CAD build for the part. Positions are in the model's coordinates, mm. A direction names the side the tool comes from. Coordinates: 2 decimals unless noted, no trailing zeros. Write each loop counter-clockwise with the first axis right and the second up, starting at its lowest first coordinate (ties: lowest second). Pieces come first, ordered by that corner, then holes. Notation, with made-up numbers: (67, 68) -> (126, 68) arc R13 cw to (126, 82) -> close; hole circle Ø10 at (26.25, -28). An arc over 180 degrees is marked (long way). Answer as CSV lines item,"result".
```python
from build123d import *

# Parameters (mm, degrees)
SKETCH1_W               = 38.1
SKETCH1_H               = 152.4
BOSS_EXTRUDE1_DEPTH     = 12.7
FILLET1_R               = 12.7
CUT_EXTRUDE1_DEPTH      = 83.55
EXTRUDE_THIN1_START     = -12.7
EXTRUDE_THIN1_DEPTH     = 12.7
CUT_EXTRUDE2_DEPTH      = 6.35
SKETCH6_W               = 35.1984056
SKETCH6_H               = 5.08
SKETCH6_R               = 1.054294776
BOSS_EXTRUDE2_DEPTH     = 5.08
CLEARANCE_1_DEPTH       = 6.35
CUT_EXTRUDE_THIN2_START = -12.7
CUT_EXTRUDE_THIN2_DEPTH = 12.7


with BuildPart() as part:
    # Sketch1 → Boss-Extrude1 (new, symmetric)
    with BuildSketch(Plane.XY):
        Rectangle(SKETCH1_W, SKETCH1_H)
    extrude(amount=BOSS_EXTRUDE1_DEPTH, both=True)

    # Fillet1
    fillet1_edges = [part.edges().sort_by_distance(p)[0] for p in [
        (19.05, -76.2, 0),
        (-19.05, -76.2, 0),
        (-19.05, 76.2, 0),
        (19.05, 76.2, 0),
    ]]
    fillet(fillet1_edges, radius=FILLET1_R)

    # Sketch2 → Cut-Extrude1 (cut, through all)
    with BuildSketch(Plane.XY.offset(12.7)):
        with BuildLine():
            Line((-17.599200768, 63.5), (-17.599200768, -63.5))
            ThreePointArc((-17.599200768, -63.5), (-14.304386146, -71.454386146), (-6.35, -74.749200768))
            Line((-6.35, -74.749200768), (6.35, -74.749200768))
            ThreePointArc((6.35, -74.749200768), (14.304386146, -71.454386146), (17.599200768, -63.5))
            Line((17.599200768, -63.5), (17.599200768, 63.5))
            ThreePointArc((17.599200768, 63.5), (14.304386146, 71.454386146), (6.35, 74.749200768))
            Line((6.35, 74.749200768), (-6.35, 74.749200768))
            ThreePointArc((-6.35, 74.749200768), (-14.304386146, 71.454386146), (-17.599200768, 63.5))
        make_face()
    extrude(amount=-CUT_EXTRUDE1_DEPTH, mode=Mode.SUBTRACT)

    # Sketch3 → Extrude-Thin1 (add)
    with BuildSketch(Plane(origin=(0, 0, -12.7), x_dir=(-1, 0, 0), z_dir=(0, 0, -1)).offset(EXTRUDE_THIN1_START)):
        with BuildLine():
            Line((-6.35, 74.749200768), (6.35, 74.749200768))
            ThreePointArc((6.35, 74.749200768), (14.304386146, 71.454386146), (17.599200768, 63.5))
            Line((17.599200768, 63.5), (17.599200768, -63.5))
            ThreePointArc((17.599200768, -63.5), (14.304386146, -71.454386146), (6.35, -74.749200768))
            Line((6.35, -74.749200768), (-6.35, -74.749200768))
            ThreePointArc((-6.35, -74.749200768), (-14.304386146, -71.454386146), (-17.599200768, -63.5))
            Line((-17.599200768, -63.5), (-17.599200768, 63.5))
            ThreePointArc((-17.599200768, 63.5), (-14.304386146, 71.454386146), (-6.35, 74.749200768))
        make_face()
        with BuildLine():
            Line((-6.35, 72.209200768), (6.35, 72.209200768))
            ThreePointArc((6.35, 72.209200768), (12.508334922, 69.658334922), (15.059200768, 63.5))
            Line((15.059200768, 63.5), (15.059200768, -63.5))
            ThreePointArc((15.059200768, -63.5), (12.508334922, -69.658334922), (6.35, -72.209200768))
            Line((6.35, -72.209200768), (-6.35, -72.209200768))
            ThreePointArc((-6.35, -72.209200768), (-12.508334922, -69.658334922), (-15.059200768, -63.5))
            Line((-15.059200768, -63.5), (-15.059200768, 63.5))
            ThreePointArc((-15.059200768, 63.5), (-12.508334922, 69.658334922), (-6.35, 72.209200768))
        make_face(mode=Mode.SUBTRACT)
    extrude(amount=EXTRUDE_THIN1_DEPTH)

    # Sketch4 → Cut-Extrude2 (cut)
    with BuildSketch(Plane(origin=(0, 0, -12.7), x_dir=(-1, 0, 0), z_dir=(0, 0, -1))):
        with BuildLine():
            Line((6.35, -76.2), (-6.35, -76.2))
            ThreePointArc((-6.35, -76.2), (-15.330256121, -72.480256121), (-19.05, -63.5))
            Line((-19.05, -63.5), (-19.05, 63.5))
            ThreePointArc((-19.05, 63.5), (-15.330256121, 72.480256121), (-6.35, 76.2))
            Line((-6.35, 76.2), (6.35, 76.2))
            ThreePointArc((6.35, 76.2), (15.330256121, 72.480256121), (19.05, 63.5))
            Line((19.05, 63.5), (19.05, -63.5))
            ThreePointArc((19.05, -63.5), (15.330256121, -72.480256121), (6.35, -76.2))
        make_face()
        with BuildLine():
            Line((-17.5992028, -63.5), (-17.5992028, 63.5))
            ThreePointArc((-17.5992028, 63.5), (-14.304387583, 71.454387583), (-6.35, 74.7492028))
            Line((-6.35, 74.7492028), (6.35, 74.7492028))
            ThreePointArc((6.35, 74.7492028), (14.304387583, 71.454387583), (17.5992028, 63.5))
            Line((17.5992028, 63.5), (17.5992028, -63.5))
            ThreePointArc((17.5992028, -63.5), (14.304387583, -71.454387583), (6.35, -74.7492028))
            Line((6.35, -74.7492028), (-6.35, -74.7492028))
            ThreePointArc((-6.35, -74.7492028), (-14.304387583, -71.454387583), (-17.5992028, -63.5))
        make_face(mode=Mode.SUBTRACT)
    extrude(amount=-CUT_EXTRUDE2_DEPTH, mode=Mode.SUBTRACT)

    # Sketch6 → Boss-Extrude2 (add)
    # profile 1 of 4: a face of its own
    with BuildSketch(Plane(origin=(0, 0, -7.62), x_dir=(-1, 0, 0), z_dir=(0, 0, -1))):
        with Locations((0, 38.431496192)):
            Rectangle(SKETCH6_W, SKETCH6_H)
        with Locations((3.015690418, 38.431496192)):
            Circle(SKETCH6_R, mode=Mode.SUBTRACT)
    # profile 2 of 4: a face of its own
    with BuildSketch(Plane(origin=(0, 0, -7.62), x_dir=(-1, 0, 0), z_dir=(0, 0, -1))):
        with Locations((0, 12.839006486)):
            Rectangle(SKETCH6_W, SKETCH6_H)
        with Locations((3.015690418, 12.839006486)):
            Circle(SKETCH6_R, mode=Mode.SUBTRACT)
    # profile 3 of 4: a face of its own
    with BuildSketch(Plane(origin=(0, 0, -7.62), x_dir=(-1, 0, 0), z_dir=(0, 0, -1))):
        with Locations((0, -12.818503808)):
            Rectangle(SKETCH6_W, SKETCH6_H)
        with Locations((3.015690418, -12.818503808)):
            Circle(SKETCH6_R, mode=Mode.SUBTRACT)
    # profile 4 of 4: a face of its own
    with BuildSketch(Plane(origin=(0, 0, -7.62), x_dir=(-1, 0, 0), z_dir=(0, 0, -1))):
        with Locations((0, -38.410993514)):
            Rectangle(SKETCH6_W, SKETCH6_H)
        with Locations((3.015690418, -38.410993514)):
            Circle(SKETCH6_R, mode=Mode.SUBTRACT)
    extrude(amount=BOSS_EXTRUDE2_DEPTH)

    # Sketch7 → Clearance 1 (cut)
    with BuildSketch(Plane(origin=(0, 0, -12.7), x_dir=(-1, 0, 0), z_dir=(0, 0, -1))):
        with BuildLine():
            Line((-17.5992028, 63.5), (-17.5992028, -63.5))
            ThreePointArc((-17.5992028, -63.5), (-14.304387583, -71.454387583), (-6.35, -74.7492028))
            Line((-6.35, -74.7492028), (6.35, -74.7492028))
            ThreePointArc((6.35, -74.7492028), (14.304387583, -71.454387583), (17.5992028, -63.5))
            Line((17.5992028, -63.5), (17.5992028, 63.5))
            ThreePointArc((17.5992028, 63.5), (14.304387583, 71.454387583), (6.35, 74.7492028))
            Line((6.35, 74.7492028), (-6.35, 74.7492028))
            ThreePointArc((-6.35, 74.7492028), (-14.304387583, 71.454387583), (-17.5992028, 63.5))
        make_face()
        with BuildLine():
            Line((-17.4722028, 63.5), (-17.4722028, -63.5))
            ThreePointArc((-17.4722028, -63.5), (-14.214585022, -71.364585022), (-6.35, -74.6222028))
            Line((-6.35, -74.6222028), (6.35, -74.6222028))
            ThreePointArc((6.35, -74.6222028), (14.214585022, -71.364585022), (17.4722028, -63.5))
            Line((17.4722028, -63.5), (17.4722028, 63.5))
            ThreePointArc((17.4722028, 63.5), (14.214585022, 71.364585022), (6.35, 74.6222028))
            Line((6.35, 74.6222028), (-6.35, 74.6222028))
            ThreePointArc((-6.35, 74.6222028), (-14.214585022, 71.364585022), (-17.4722028, 63.5))
        make_face(mode=Mode.SUBTRACT)
    extrude(amount=-CLEARANCE_1_DEPTH, mode=Mode.SUBTRACT)

    # Sketch8 → Cut-Extrude-Thin2 (cut)
    with BuildSketch(Plane.XY.offset(12.7).offset(CUT_EXTRUDE_THIN2_START)):
        with BuildLine():
            Line((-17.726200768, 63.5), (-17.726200768, -63.5))
            ThreePointArc((-17.726200768, -63.5), (-14.394188707, -71.544188707), (-6.35, -74.876200768))
            Line((-6.35, -74.876200768), (6.35, -74.876200768))
            ThreePointArc((6.35, -74.876200768), (14.394188707, -71.544188707), (17.726200768, -63.5))
            Line((17.726200768, -63.5), (17.726200768, 63.5))
            ThreePointArc((17.726200768, 63.5), (14.394188707, 71.544188707), (6.35, 74.876200768))
            Line((6.35, 74.876200768), (-6.35, 74.876200768))
            ThreePointArc((-6.35, 74.876200768), (-14.394188707, 71.544188707), (-17.726200768, 63.5))
        make_face()
        with BuildLine():
            Line((-17.599200768, 63.5), (-17.599200768, -63.5))
            ThreePointArc((-17.599200768, -63.5), (-14.304386146, -71.454386146), (-6.35, -74.749200768))
            Line((-6.35, -74.749200768), (6.35, -74.749200768))
            ThreePointArc((6.35, -74.749200768), (14.304386146, -71.454386146), (17.599200768, -63.5))
            Line((17.599200768, -63.5), (17.599200768, 63.5))
            ThreePointArc((17.599200768, 63.5), (14.304386146, 71.454386146), (6.35, 74.749200768))
            Line((6.35, 74.749200768), (-6.35, 74.749200768))
            ThreePointArc((-6.35, 74.749200768), (-14.304386146, 71.454386146), (-17.599200768, 63.5))
        make_face(mode=Mode.SUBTRACT)
    extrude(amount=CUT_EXTRUDE_THIN2_DEPTH, mode=Mode.SUBTRACT)


solid = part.part
```
Item 1: 3-axis set-ups, long thin cutter, end or side, ignore diameter. For faces 1 (the flat face through (17.726, -1, 6)), 2 (the flat face through (0, 10.299, -10)), 3 (the flat face through (17.472, 1, -10)): which of +Z, -Z, +X, -X, +Y, -Y reach the whole face in a straight line?
Answer below:
face 1,"+Z"
face 2,"+Z, -Z"
face 3,"-Z, +X, +Y, -Y"
Item 2: Wall check: line 1 (Y direction, x = 7, z = -9.75); line 2 (Y direction, x = -4, z = 2); line 3 (X direction, y = 60.5, z = 4.25). Give the ranges that are in metal, low to high. Write a range as from..to.
Answer below:
line 1,"y = -74.6..-72.18, -40.95..-35.87, -15.36..-10.28, 10.3..15.38, 35.89..40.97, 72.18..74.6"
line 2,"y = -76.2..-74.88, 74.88..76.2"
line 3,"x = -19.05..-17.73, 17.73..19.05"
Item 3: Saw through at D-D on z = -1.5. Give the cut face in (x, y), and give its area (3 significant figures).
Answer below:
outline,"(-19.05, -63.5) arc R12.7 ccw to (-6.35, -76.2) -> (6.35, -76.2) arc R12.7 ccw to (19.05, -63.5) -> (19.05, 63.5) arc R12.7 ccw to (6.35, 76.2) -> (-6.35, 76.2) arc R12.7 ccw to (-19.05, 63.5) -> close; hole (-15.06, -63.5) arc R8.71 ccw to (-6.35, -72.21) -> (6.35, -72.21) arc R8.71 ccw to (15.06, -63.5) -> (15.06, 63.5) arc R8.71 ccw to (6.35, 72.21) -> (-6.35, 72.21) arc R8.71 ccw to (-15.06, 63.5) -> close"
area,"1,380 mm2"
Item 4: Saw through at B-B on x = -0.5. State how many separate pieces and enclosed holes the cut face has, and give its area (3 significant figures).
Answer below:
separate pieces,"6"
enclosed holes,"0"
area,"218 mm2"
Item 5: Saw through at C-C on z = 6.75. Give the cut face in (x, y), and give its area (3 significant figures).
Answer below:
outline,"(-19.05, -63.5) arc R12.7 ccw to (-6.35, -76.2) -> (6.35, -76.2) arc R12.7 ccw to (19.05, -63.5) -> (19.05, 63.5) arc R12.7 ccw to (6.35, 76.2) -> (-6.35, 76.2) arc R12.7 ccw to (-19.05, 63.5) -> close; hole (-17.73, -63.5) arc R11.38 ccw to (-6.35, -74.88) -> (6.35, -74.88) arc R11.38 ccw to (17.73, -63.5) -> (17.73, 63.5) arc R11.38 ccw to (6.35, 74.88) -> (-6.35, 74.88) arc R11.38 ccw to (-17.73, 63.5) -> close"
area,"470 mm2"
Item 6: Saw through at A-A on y = 46. Give the cut face in (x, z).
Answer below:
outline,"(-19.05, -6.35) -> (-17.47, -6.35) -> (-17.47, -12.7) -> (-15.06, -12.7) -> (-15.06, 0) -> (-17.73, 0) -> (-17.73, 12.7) -> (-19.05, 12.7) -> close; (15.06, -12.7) -> (17.47, -12.7) -> (17.47, -6.35) -> (19.05, -6.35) -> (19.05, 12.7) -> (17.73, 12.7) -> (17.73, 0) -> (15.06, 0) -> close"
Item 7: Flat gauge pins, fed straight in: pin 1 (2.5 mm diameter, centred on x = -6.5, z = -10.5, fed in from -Y); pin 2 (4 mm diameter, centred on x = 12, z = -8, fed in from -Y); pin 3 (1.9 mm diameter, centred on y = 5.5, z = -9, fed in from -X). Where does each tip first touch, or does it go through?
Answer below:
pin 1,"stops at y = -74.62"
pin 2,"stops at y = -75.37"
pin 3,"stops at x = -17.47"
Item 8: Two-plate mould, pull along Y, no slides. Class faces 4 (the cylindrical face through (-14.13, -71.45, -9.57)), 5 (the flat face through (18, 0, -6.35)), 6 (the cylindrical face through (-14.31, 71.63, 6.26)): pulls with the +Y half, pulls with the -Y half, needs draft (parallel to the pull), parting line crosses it, or undercut.
Answer below:
face 4,"pulls with the -Y half"
face 5,"needs draft"
face 6,"undercut"
